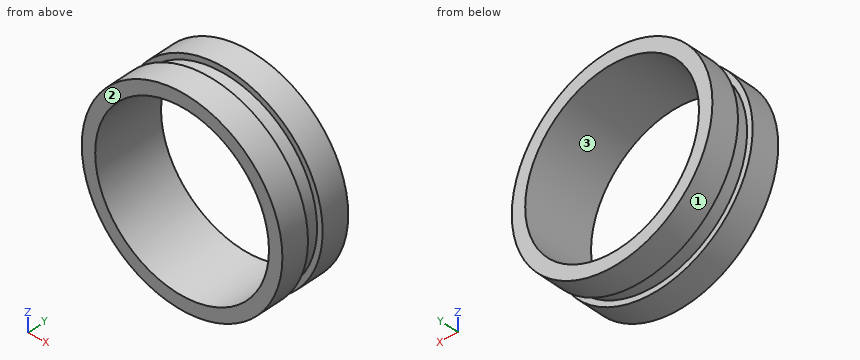
```python
from build123d import *

# Parameters (mm, degrees)
F0_R     = 12
F1_DEPTH = 9
F2_R     = 12.7
F3_DEPTH = 3.5
F4_R     = 12.7
F4_R_2   = 12
F5_DEPTH = 3.5
F6_D     = 22


# Not quite as in the source:
# - a feature names something its author has since deleted; it is built from what else it names


with BuildPart() as f1:
    # F0 (on Front) → F1 (new body)
    with BuildSketch(Plane.XZ):
        with Locations((-29.9285538495, 19.7017099708)):
            Circle(F0_R)
    extrude(amount=F1_DEPTH)

    # F2 (on Front) → F3 (join)
    with BuildSketch(Plane.XZ):
        with Locations((-29.9285538495, 19.7017099708)):
            Circle(F2_R)
    extrude(amount=F3_DEPTH)

    # F4 (on face) → F5 (join)
    with BuildSketch(Plane.XZ.offset(9)):
        with Locations((-29.9285538495, 19.7017099708)):
            Circle(F4_R)
        with Locations((-29.9285538495, 19.7017099708)):
            Circle(F4_R_2, mode=Mode.SUBTRACT)
    extrude(amount=-F5_DEPTH)

    # F6 (through all)
    with Locations(Plane(origin=(0, 0, 0), x_dir=(1, 0, 0), z_dir=(0, 1, 0))):
        with Locations((-29.9285538495, -19.7017099708)):
            Hole(F6_D / 2)


solid = f1.part
```
The listing builds one solid part. Answer for the finished solid, in the listing's coordinates (mm). Face numbers are marked on the shaded views. Round coordinates to 2 decimals unless told otherwise and drop trailing zeros. Write each loop counter-clockwise with the first axis right and the second up, starting at its lowest first coordinate (ties: lowest second). Pieces come first, ordered by that corner, then holes. Notation, with made-up numbers: (-29.75, -5.75) -> (-23.75, -5.75) arc R26 cw to (-23.75, 27.25) -> close; hole circle Ø1 at (-35.75, 80). An arc over 180 degrees is marked (long way). Answer as a JSON object with one key per item and string values. Group by question number.
Q1. Each of these flat-tipped pins is pushed along its axis until it touches: pin 1 Ø12.5 at (x, z) = (-35.5, 23) entering from +Y; pin 2 Ø1.5 at (x, y) = (-35, -6.5) entering from +Z; pin 3 Ø5 at (x, y) = (-36, -8) entering from +Z. Where does it stop, or does it pass through?
Q2. Section A-A (z = 21) is taken. Write down the section's boundary in (x, y).
Q3. Section C-C (y = -4) is taken. Write down the section's boundary in (x, z).
Q4. Determine the mould class of the marked faces 1, 2 and 3 for opening direction Z: pulls with the +Z half, pulls with the -Z half, needs draft (parallel to the pull), parting line crosses it, or undercut.
Q5. Straight lines are drawn through the part: line 1 along Y through (x, z) = (-24.75, 8.75); line 2 along X through (y, z) = (-2.75, 20); line 3 along Z through (x, y) = (-21.75, -2.5). For each, find the intervals that lie inside material, in ascending order.
Q6. Section D-D (y = -8.5) is taken. Write down the section's boundary in (x, z).
Q7. Section B-B (x = -32.75) is taken. Write down the section's boundary in (y, z).
Check values:
{
 "1": {"pin 1": "y = 0", "pin 2": "z = 31.64", "pin 3": "z = 31.89"},
 "2": {"outline": "(-42.56, -9) -> (-40.85, -9) -> (-40.85, 0) -> (-42.56, 0) -> (-42.56, -3.5) -> (-41.86, -3.5) -> (-41.86, -5.5) -> (-42.56, -5.5) -> close; (-19.01, -9) -> (-17.3, -9) -> (-17.3, -5.5) -> (-18, -5.5) -> (-18, -3.5) -> (-17.3, -3.5) -> (-17.3, 0) -> (-19.01, 0) -> close"},
 "3": {"outline": "circle Ø24 at (-29.93, 19.7); hole circle Ø22 at (-29.93, 19.7)"},
 "4": {"face 1": "parting line crosses it", "face 2": "needs draft", "face 3": "undercut"},
 "5": {"line 1": "-9 to -5.5, -3.5 to 0", "line 2": "-42.63 to -40.92, -18.93 to -17.23", "line 3": "9.99 to 12.35, 27.06 to 29.42"},
 "6": {"outline": "circle Ø25.4 at (-29.93, 19.7); hole circle Ø22 at (-29.93, 19.7)"},
 "7": {"outline": "(-9, 7.32) -> (-5.5, 7.32) -> (-5.5, 8.04) -> (-3.5, 8.04) -> (-3.5, 7.32) -> (0, 7.32) -> (0, 9.07) -> (-9, 9.07) -> close; (-9, 30.33) -> (0, 30.33) -> (0, 32.08) -> (-3.5, 32.08) -> (-3.5, 31.37) -> (-5.5, 31.37) -> (-5.5, 32.08) -> (-9, 32.08) -> close"}
}
